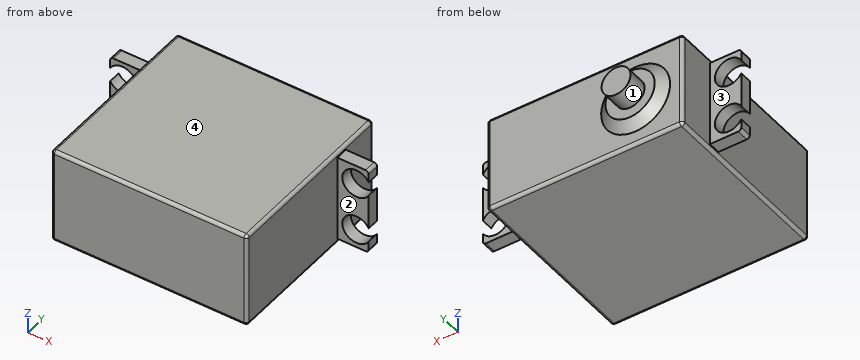
from build123d import *

# Parameters (mm, degrees)
BODY_W                      = 40.386
BODY_H                      = 19.812
SERVO_BODY_DEPTH            = 37.592
TAB_W                       = 17.907
TAB_H                       = 2.54
MOUNTING_TAB_DEPTH          = 6.477
FILLET1_R                   = 0.635
HOLES_R                     = 2.921
MOUNTING_HOLES_DEPTH        = 41.957844572
FILLET1_OF_MOUNTING_TAB_2_R = 0.635
SHAFT_R                     = 2.9845
SPLINE_SHAFT_DEPTH          = 4.191
FILLET2_R                   = 0.635


with BuildPart() as part:
    # body → servo_body (new body)
    with BuildSketch(Plane(origin=(0, 0, 0), x_dir=(1, 0, 0), z_dir=(0, 1, 0))):
        Rectangle(BODY_W, BODY_H)
    extrude(amount=SERVO_BODY_DEPTH)

    # tab → mounting_tab (add)
    with BuildSketch(Plane.ZY.offset(20.193)):
        with Locations((0, 28.194)):
            Rectangle(TAB_W, TAB_H)
    mounting_tab = extrude(amount=MOUNTING_TAB_DEPTH)

    # Fillet1
    fillet1_edges = [part.edges().sort_by_distance(p)[0] for p in [
        (-26.67, 28.194, -8.9535),
        (-26.67, 28.194, 8.9535),
    ]]
    fillet(fillet1_edges, radius=FILLET1_R)

    # holes → mounting_holes (cut, through all)
    with BuildSketch(Plane(origin=(0, 29.464, 0), x_dir=(-1, 0, 0), z_dir=(0, 1, 0))):
        with Locations((24.13, -5.08)):
            Circle(HOLES_R)
        with Locations((24.13, 5.08)):
            Circle(HOLES_R)
    mounting_holes = extrude(amount=-MOUNTING_HOLES_DEPTH, mode=Mode.SUBTRACT)

    # mounting_tab_2: mounting_tab, mounting_holes across plane
    add(mounting_tab.mirror(Plane(origin=(0, 0, 0), x_dir=(0, 0, 1), z_dir=(1, 0, 0))))
    add(mounting_holes.mirror(Plane(origin=(0, 0, 0), x_dir=(0, 0, 1), z_dir=(1, 0, 0))), mode=Mode.SUBTRACT)

    # Fillet1 of mounting_tab_2
    fillet1_of_mounting_tab_2_edges = [part.edges().sort_by_distance(p)[0] for p in [
        (26.67, 28.194, -8.9535),
        (26.67, 28.194, 8.9535),
    ]]
    fillet(fillet1_of_mounting_tab_2_edges, radius=FILLET1_OF_MOUNTING_TAB_2_R)

    # Sketch4 → Boss-Revolve1 (revolve)
    with BuildSketch(Plane.XY, mode=Mode.PRIVATE) as boss_revolve1_sk:
        Polygon((-10.4902, 37.592), (-3.3782, 37.592), (-5.4102, 39.243), (-10.4902, 39.243), align=None)
    revolve(boss_revolve1_sk.sketch.rotate(Axis((-10.4902, 39.598741813, 0), (0, -1, 0)), 90), axis=Axis((-10.4902, 39.598741813, 0), (0, -1, 0)))

    # shaft → spline_shaft (add)
    with BuildSketch(Plane(origin=(0, 39.243, 0), x_dir=(-1, 0, 0), z_dir=(0, 1, 0))):
        with Locations(Location((10.4902, 0, 0), (0, 0, 270))):
            Circle(SHAFT_R)
    extrude(amount=SPLINE_SHAFT_DEPTH)

    # Fillet2
    fillet2_edges = [part.edges().sort_by_distance(p)[0] for p in [
        (20.193, 37.592, 0),
        (0, 37.592, -9.906),
        (-20.193, 37.592, 0),
        (0, 0, -9.906),
        (20.193, 0, 0),
        (0, 0, 9.906),
        (-20.193, 0, 0),
        (0, 37.592, 9.906),
        (-20.193, 18.796, -9.906),
        (20.193, 18.796, -9.906),
        (20.193, 18.796, 9.906),
        (-20.193, 18.796, 9.906),
    ]]
    fillet(fillet2_edges, radius=FILLET2_R)


solid = part.part
Verification items for the finished model (mm, model axes). Face numbers are marked on the shaded views. A direction names the side the tool comes from. Coordinates: 2 decimals unless noted, no trailing zeros. Order: outer loops, then holes, each group sorted by start corner. A loop starts at its lowest first (then second) coordinate and runs counter-clockwise, first axis right, second up. Notation, with made-up numbers: M 51.5,47 L 81.5,47 A32 cw 81.5,86 Z; hole C 59.5,-9.75 d8. An arc over 180 degrees is marked long. Return JSON: item names as keys, results as strings.
1) Access from +Z, -Z, +X, -X, +Y, -Y to the whole of each face (thin tool, end or side, straight path). Record for the marked faces 1, 2, 3 and 4.
Answer list:
{"face 1": "+Y", "face 2": "+Z, -Z, +X, -Y", "face 3": "+Z, -Z, -X, +Y", "face 4": "+Z, +X, -X, +Y, -Y"}
2) Cross-section at A-A, the plane x = -24.13. Record the boundary of the cut face in (y, z).
Answer list:
{"outline": "M 26.92,-8.95 L 29.46,-8.95 L 29.46,-8 L 26.92,-8 Z; M 26.92,-2.16 L 29.46,-2.16 L 29.46,2.16 L 26.92,2.16 Z; M 26.92,8 L 29.46,8 L 29.46,8.95 L 26.92,8.95 Z"}
3) Cross-section at C-C, the plane z = 0. Record the boundary of the cut face in (x, y) (3 decimals).
Answer list:
{"outline": "M -26.67,26.924 L -20.193,26.924 L -20.193,0.635 A0.635 ccw -19.558,0 L 19.558,0 A0.635 ccw 20.193,0.635 L 20.193,26.924 L 26.67,26.924 L 26.67,29.464 L 20.193,29.464 L 20.193,36.957 A0.635 ccw 19.558,37.592 L -3.378,37.592 L -5.41,39.243 L -7.506,39.243 L -7.506,43.434 L -13.475,43.434 L -13.475,39.243 L -15.57,39.243 L -17.602,37.592 L -19.558,37.592 A0.635 ccw -20.193,36.957 L -20.193,29.464 L -26.67,29.464 Z"}
4) Gauge pin test, flat ends, axial feed: pin 1 (0.8 mm diameter, centred on x = 23.5, y = 28, fed in from -Z); pin 2 (3 mm diameter, centred on x = 22, y = 28, fed in from +Z); pin 3 (1.9 mm diameter, centred on x = 23, z = 4, fed in from +Y); pin 4 (9.5 mm diameter, centred on y = 16.5, z = -2.5, fed in from +X). Record the tip position at first contact, or that the pin passes through.
Answer list:
{"pin 1": "z = -8.95", "pin 2": "z = 8.95", "pin 3": "through", "pin 4": "x = 20.19"}
5) Cross-section at D-D, the plane x = 13.5. Record the boundary of the cut face in (y, z) (3 decimals), and give its area (3 significant figures).
Answer list:
{"outline": "M 0,-9.271 A0.635 ccw 0.635,-9.906 L 36.957,-9.906 A0.635 ccw 37.592,-9.271 L 37.592,9.271 A0.635 ccw 36.957,9.906 L 0.635,9.906 A0.635 ccw 0,9.271 Z", "area": "744 mm2"}
6) Thickness scan on L1, parallel to Z at x = 24.13, y = 27.7; L2, parallel to Y at x = 12.5, z = 8; L3, parallel to Y at x = 20.5, z = -6.5. Record the ranges inside material, lowest first. Write a range as [from, to].
Answer list:
{"L1": "[-8.95, -8], [-2.16, 2.16], [8, 8.95]", "L2": "[0, 37.59]", "L3": "[26.92, 29.46]"}
